Part model, mm, in its own coordinate system. A direction names the side the tool comes from. Coordinates: 2 decimals unless noted, no trailing zeros. Loops run counter-clockwise (first coordinate to the right, second up) from the corner with the lowest first, then second, coordinate; pieces in that order, holes last. Notation, with made-up numbers: M -12.75,23 L 0.25,23 A24 ccw 0.25,43 Z; hole C 8,55 d3. An arc over 180 degrees is marked long. Use a Markdown table: item, result. Add a question column.
1) Tool access for faces 4 (the flat face through (-12, 7.4, 1)), 5 (the flat face through (0, 3, 0)), 6 (the cylindrical face through (-15.7, 3, 1)): list every direction of +Z, -Z, +X, -X, +Y, -Y with a clear straight run to the whole face (end or side of a thin tool).
2) Band-saw the part on C-C (y = -3.05). List the corners of the cut face in (x, z), plus the area to 3 significant figures.
3) Band-saw the part on D-D (z = 0.45). List the corners of the cut face in (x, y).
4) Band-saw the part on B-B (y = 0). List the corners of the cut face in (x, z).
5) Pin check, flat tips, straight feed: pin 1 Ø1 at (x, z) = (-13.5, 1) entering from +Y; pin 2 Ø0.6 at (y, z) = (8.5, 0.5) entering from +X. Stop position of each tip, or through.
6) Wall check: probe 1 along Y at (x, z) = (0, 0.25); probe 2 along X at (y, z) = (2.75, 0.45); probe 3 along X at (y, z) = (8, 1.05). Give the ranges that are in metal, low to high. Write a range as from..to.
7) Pull direction Y, two halves, no side cores. Call faces 1 (the flat face through (0, -7.4, 1)), 2 (the flat face through (0, 9.5, 1)), 3 (the flat face through (13, 4.1, 1)): released by +Y, released by -Y, zero draft, split by the parting line, or undercut.
8) Band-saw the part on A-A (x = 0). List the corners of the cut face in (y, z).
from build123d import *

# Parameters (mm, degrees)
SKETCH_1_R      = 1.55
EXTRUDE_1_DEPTH = 2.1


with BuildPart() as part:
    # 草图1 → 凸台-拉伸1 (new body)
    with BuildSketch(Plane.XY):
        with BuildLine():
            Line((-17.5, -7.4), (17.5, -7.4))
            Line((17.5, -7.4), (17.5, 7.4))
            Line((17.5, 7.4), (7.1, 7.4))
            ThreePointArc((7.1, 7.4), (6.05, 6.35), (5, 7.4))
            Line((5, 7.4), (5, 9.5))
            Line((5, 9.5), (-5, 9.5))
            Line((-5, 9.5), (-5, 7.4))
            ThreePointArc((-5, 7.4), (-6.05, 6.35), (-7.1, 7.4))
            Line((-7.1, 7.4), (-17.5, 7.4))
            Line((-17.5, 7.4), (-17.5, -7.4))
        make_face()
        with BuildLine():
            Line((-12.35, -4.1), (-14.65, -4.1))
            ThreePointArc((-14.65, -4.1), (-15.7, -3.05), (-14.65, -2))
            Line((-14.65, -2), (-14.65, 2))
            ThreePointArc((-14.65, 2), (-15.7, 3.05), (-14.65, 4.1))
            Line((-14.65, 4.1), (-12.35, 4.1))
            ThreePointArc((-12.35, 4.1), (-11.3, 3.05), (-12.35, 2))
            Line((-12.35, 2), (-12.35, -2))
            ThreePointArc((-12.35, -2), (-11.3, -3.05), (-12.35, -4.1))
        make_face(mode=Mode.SUBTRACT)
        Circle(SKETCH_1_R, mode=Mode.SUBTRACT)
        with BuildLine():
            ThreePointArc((12.35, 2), (11.3, 3.05), (12.35, 4.1))
            Line((12.35, 4.1), (14.65, 4.1))
            ThreePointArc((14.65, 4.1), (15.7, 3.05), (14.65, 2))
            Line((14.65, 2), (14.65, -2))
            ThreePointArc((14.65, -2), (15.7, -3.05), (14.65, -4.1))
            Line((14.65, -4.1), (12.35, -4.1))
            ThreePointArc((12.35, -4.1), (11.3, -3.05), (12.35, -2))
            Line((12.35, -2), (12.35, 2))
        make_face(mode=Mode.SUBTRACT)
    extrude(amount=EXTRUDE_1_DEPTH)


solid = part.part
Entries:
| question | item | result |
|---|---|---|
| 1 | face 4 | +Z, -Z, -X, +Y |
| 1 | face 5 | -Z, +X, -X, +Y, -Y |
| 1 | face 6 | +Z, -Z |
| 2 | outline | M -17.5,0 L -15.7,0 L -15.7,2.1 L -17.5,2.1 Z; M -11.3,0 L 11.3,0 L 11.3,2.1 L -11.3,2.1 Z; M 15.7,0 L 17.5,0 L 17.5,2.1 L 15.7,2.1 Z |
| 2 | area | 55.0 mm2 |
| 3 | outline | M -17.5,-7.4 L 17.5,-7.4 L 17.5,7.4 L 7.1,7.4 A1.05 cw 5,7.4 L 5,9.5 L -5,9.5 L -5,7.4 A1.05 cw -7.1,7.4 L -17.5,7.4 Z; hole M -14.65,-4.1 L -12.35,-4.1 A1.05 ccw -12.35,-2 L -12.35,2 A1.05 ccw -12.35,4.1 L -14.65,4.1 A1.05 ccw -14.65,2 L -14.65,-2 A1.05 ccw Z; hole C 0,0 d3.1; hole M 12.35,-4.1 L 14.65,-4.1 A1.05 ccw 14.65,-2 L 14.65,2 A1.05 ccw 14.65,4.1 L 12.35,4.1 A1.05 ccw 12.35,2 L 12.35,-2 A1.05 ccw Z |
| 4 | outline | M -17.5,0 L -14.65,0 L -14.65,2.1 L -17.5,2.1 Z; M -12.35,0 L -1.55,0 L -1.55,2.1 L -12.35,2.1 Z; M 1.55,0 L 12.35,0 L 12.35,2.1 L 1.55,2.1 Z; M 14.65,0 L 17.5,0 L 17.5,2.1 L 14.65,2.1 Z |
| 5 | pin 1 | y = 7.4 |
| 5 | pin 2 | x = 5 |
| 6 | probe 1 | -7.4..-1.55, 1.55..9.5 |
| 6 | probe 2 | -17.5..-15.66, -11.34..11.34, 15.66..17.5 |
| 6 | probe 3 | -5..5 |
| 7 | face 1 | released by -Y |
| 7 | face 2 | released by +Y |
| 7 | face 3 | undercut |
| 8 | outline | M -7.4,0 L -1.55,0 L -1.55,2.1 L -7.4,2.1 Z; M 1.55,0 L 9.5,0 L 9.5,2.1 L 1.55,2.1 Z |
